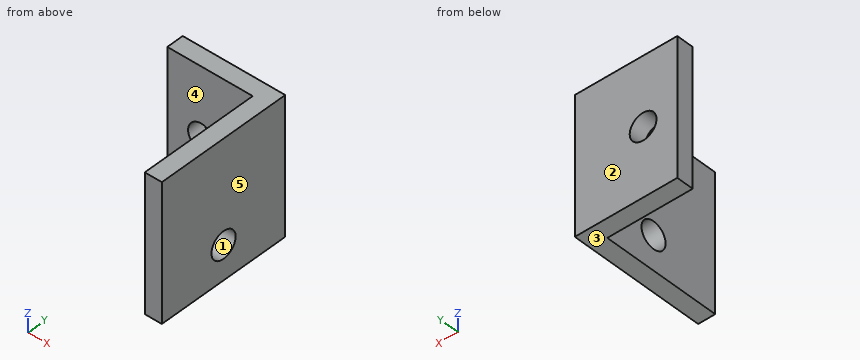
```python
from build123d import *

# Parameters (mm, degrees)
EXTRUDE_THIN1_DEPTH            = 25.4
F_9_0_196_DIAMETER_HOLE1_D     = 4.9784
F_9_0_196_DIAMETER_HOLE1_DEPTH = 3.175
F_9_0_196_DIAMETER_HOLE3_D     = 4.9784
F_9_0_196_DIAMETER_HOLE3_DEPTH = 3.175
SKETCH11_W                     = 25.4
SKETCH11_H                     = 3.175
CUT_EXTRUDE1_DEPTH             = 6.35


with BuildPart() as part:
    # Sketch1 → Extrude-Thin1 (new body)
    with BuildSketch(Plane.XY):
        Polygon((-524.51, -25.4), (-524.51, 0), (-549.91, 0), (-549.91, -3.175), (-527.685, -3.175), (-527.685, -25.4), align=None)
    extrude(amount=-EXTRUDE_THIN1_DEPTH)

    # #9 (0.196) Diameter Hole1
    with Locations(Plane.ZY.offset(527.685)):
        with Locations((-19.05, -12.7)):
            Hole(F_9_0_196_DIAMETER_HOLE1_D / 2, depth=F_9_0_196_DIAMETER_HOLE1_DEPTH)

    # #9 (0.196) Diameter Hole3
    with Locations(Plane(origin=(0, -3.175, 0), x_dir=(-1, 0, 0), z_dir=(0, -1, 0))):
        with Locations((537.21, 12.7)):
            Hole(F_9_0_196_DIAMETER_HOLE3_D / 2, depth=F_9_0_196_DIAMETER_HOLE3_DEPTH)

    # Sketch11 → Cut-Extrude1 (cut)
    with BuildSketch(Plane.ZY.offset(549.91)):
        with Locations((-12.7, -1.5875)):
            Rectangle(SKETCH11_W, SKETCH11_H)
    extrude(amount=-CUT_EXTRUDE1_DEPTH, mode=Mode.SUBTRACT)


solid = part.part
```
The listing builds one solid part. Answer for the finished solid, in the listing's coordinates (mm). Face numbers are marked on the shaded views. A direction names the side the tool comes from. Give positions to 0.01 mm unless a question says otherwise; leave off trailing zeros. Order: outer loops, then holes, each group sorted by start corner. A loop starts at its lowest first (then second) coordinate and runs counter-clockwise, first axis right, second up.
1) Determine the mould class of the marked faces 1, 2 and 3 for opening direction Z: pulls with the +Z half, pulls with the -Z half, needs draft (parallel to the pull), parting line crosses it, or undercut.
Reported:
face 1: undercut
face 2: needs draft
face 3: pulls with the -Z half
2) Find section C-C on x = -537.21. Write down the section's boundary in (y, z) (3 decimals).
Reported:
outline: (-3.175, -25.4) - (0, -25.4) - (0, -15.189) - (-3.175, -15.189) - close; (-3.175, -10.211) - (0, -10.211) - (0, 0) - (-3.175, 0) - close
3) Find section A-A on z = -12.7. Write down the section's boundary in (x, y) (3 decimals), then the cut area to 3 significant figures.
Reported:
outline: (-543.56, -3.175) - (-539.699, -3.175) - (-539.699, 0) - (-543.56, 0) - close; (-534.721, -3.175) - (-527.685, -3.175) - (-527.685, -25.4) - (-524.51, -25.4) - (-524.51, 0) - (-534.721, 0) - close
area: 115 mm2
4) Find section B-B on y = -12.7. Write down the section's boundary in (x, z) (3 decimals), then the cut area to 3 significant figures.
Reported:
outline: (-527.685, -25.4) - (-524.51, -25.4) - (-524.51, -21.539) - (-527.685, -21.539) - close; (-527.685, -16.561) - (-524.51, -16.561) - (-524.51, 0) - (-527.685, 0) - close
area: 64.8 mm2
5) Find section D-D on x = -526. Write down the section's boundary in (y, z).
Reported:
outline: (-25.4, -25.4) - (0, -25.4) - (0, 0) - (-25.4, 0) - close; hole circle Ø4.98 at (-12.7, -19.05)
6) Given P1, Ø1, axis at x = -531.5, z = -12.5, coming from the -Y side (3 decimals); P2, Ø6.5, axis at y = -17.5, z = -12, coming from the -X side (3 decimals), each flat-ended and moving along its own axis, determine where each tip first touches the part or whether it passes through.
Reported:
P1: stops at y = -3.175
P2: stops at x = -527.685
7) For the marked faces 4 and 5, determine the directions among +Z, -Z, +X, -X, +Y, -Y from which every point of the face is accessible in a straight line to the end or side of a thin tool.
Reported:
face 4: +Z, -Z, -X, -Y
face 5: +Z, -Z, +X, +Y, -Y
8) Consider line 1 along X through (y, z) = (-2.45, -12.7); line 2 along Z through (x, y) = (-537.21, -1.85); line 3 along Y through (x, z) = (-532.25, -18.75) (3 decimals). Determine where each line is inside the solid, lowest interval first.
Reported:
line 1: x = -543.56 to -539.7, -534.72 to -524.51
line 2: z = -25.4 to -15.19, -10.21 to 0
line 3: y = -3.175 to 0
